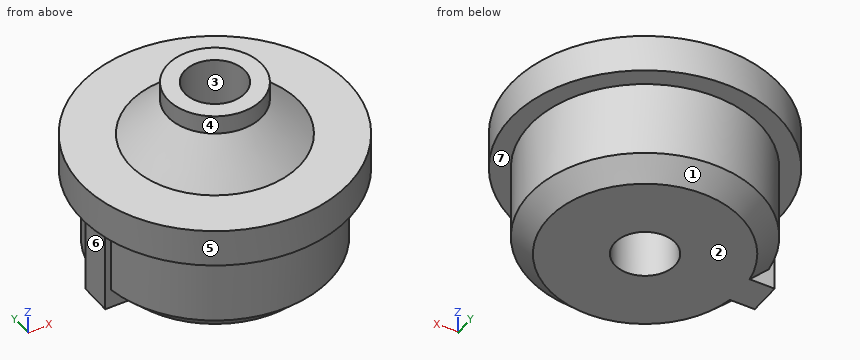
```python
from build123d import *

# Parameters (mm, degrees)
EXTRUDE_1_DEPTH     = 5
SKETCH_2_R          = 7.1
EXTRUDE_2_DEPTH     = 2
SKETCH_3_R          = 2.5
EXTRUDE_3_DEPTH     = 7
CHAMFER_1_SIZE      = 2
SKETCH_4_R          = 1.6
CUT_EXTRUDE_1_DEPTH = 30
CHAMFER_2_SIZE      = 1
MOVE_FACE_1_BY      = 4


with BuildPart() as part:
    # ｽｹｯﾁ1 → ﾎﾞｽ - 押し出し1 (new body)
    with BuildSketch(Plane.XY):
        with BuildLine():
            Line((-6.35, -0.875), (-6.036917674, -0.875))
            ThreePointArc((-6.036917674, -0.875), (6.1, 0), (-6.036917674, 0.875))
            Line((-6.036917674, 0.875), (-6.35, 0.875))
            Line((-6.35, 0.875), (-6.35, -0.875))
        make_face()
    extrude(amount=-EXTRUDE_1_DEPTH)

    # ｽｹｯﾁ2 → ﾎﾞｽ - 押し出し2 (add)
    with BuildSketch(Plane.XY):
        Circle(SKETCH_2_R)
    extrude(amount=EXTRUDE_2_DEPTH)

    # ｽｹｯﾁ3 → ﾎﾞｽ - 押し出し3 (add)
    with BuildSketch(Plane.XY.offset(2)):
        Circle(SKETCH_3_R)
    extrude(amount=EXTRUDE_3_DEPTH)

    # 面取り1
    chamfer_1_edges = [part.edges().sort_by_distance(p)[0] for p in [
        (-2.5, 0, 2),
    ]]
    chamfer(chamfer_1_edges, length=CHAMFER_1_SIZE)

    # ｽｹｯﾁ4 → ｶｯﾄ - 押し出し1 (cut)
    with BuildSketch(Plane.XY.offset(9)):
        Circle(SKETCH_4_R)
    extrude(amount=-CUT_EXTRUDE_1_DEPTH, mode=Mode.SUBTRACT)

    # 面取り2
    chamfer_2_edges = [part.edges().sort_by_distance(p)[0] for p in [
        (6.1, 0, -5),
    ]]
    chamfer(chamfer_2_edges, length=CHAMFER_2_SIZE)

    # Move Face 1: a face moved inward by 4.0
    extrude(part.faces().sort_by_distance((0, -2, 9))[0], amount=MOVE_FACE_1_BY, dir=(0, 0, -1), mode=Mode.SUBTRACT)


solid = part.part
```
Check sheet for the modelled part. Datum: model origin and axes. Units: mm. Face numbers are marked on the shaded views. A direction names the side the tool comes from. Give positions to 0.01 mm unless a question says otherwise; leave off trailing zeros. Order: outer loops, then holes, each group sorted by start corner. A loop starts at its lowest first (then second) coordinate and runs counter-clockwise, first axis right, second up. Notation, with made-up numbers: (53.25, -37) -> (60.25, -37) arc R28 ccw to (60.25, -6) -> close; hole circle Ø5 at (15, 46.25). An arc over 180 degrees is marked (long way). Return JSON: item names as keys, results as strings.
1. Cross-section at C-C, the plane z = 3.5. Record the cut outline in (x, y).
From the geometry:
{"outline": "circle Ø6 at (0, 0); hole circle Ø3.2 at (0, 0)"}
2. Material ranges on probe 1 along Y at (x, z) = (0, -2.75); probe 2 along Y at (x, z) = (-5.75, -4.5) (3 decimals); probe 3 along Z at (x, y) = (-0.5, -5), recorded low to high. Write a range as [from, to].
From the geometry:
{"probe 1": "[-6.1, -1.6], [1.6, 6.1]", "probe 2": "[-0.875, 0.875]", "probe 3": "[-5, 2]"}
3. Cross-section at A-A, the plane y = 0. Record the cut outline in (x, z), plus the area to 4 significant figures.
From the geometry:
{"outline": "(-7.1, 0) -> (-6.35, 0) -> (-6.35, -5) -> (-1.6, -5) -> (-1.6, 5) -> (-2.5, 5) -> (-2.5, 4) -> (-4.5, 2) -> (-7.1, 2) -> close; (1.6, -5) -> (5.1, -5) -> (6.1, -4) -> (6.1, 0) -> (7.1, 0) -> (7.1, 2) -> (4.5, 2) -> (2.5, 4) -> (2.5, 5) -> (1.6, 5) -> close", "area": "77.15 mm^2"}
4. Cross-section at B-B, the plane x = 0. Record the cut outline in (y, z), plus the area to 3 significant figures.
From the geometry:
{"outline": "(-7.1, 0) -> (-6.1, 0) -> (-6.1, -4) -> (-5.1, -5) -> (-1.6, -5) -> (-1.6, 5) -> (-2.5, 5) -> (-2.5, 4) -> (-4.5, 2) -> (-7.1, 2) -> close; (1.6, -5) -> (5.1, -5) -> (6.1, -4) -> (6.1, 0) -> (7.1, 0) -> (7.1, 2) -> (4.5, 2) -> (2.5, 4) -> (2.5, 5) -> (1.6, 5) -> close", "area": "75.4 mm^2"}
5. Set-up check for the marked faces 4, 5, 6 and 7: record each of +Z, -Z, +X, -X, +Y, -Y from which the full face is reachable in a straight line by a thin tool's end or side.
From the geometry:
{"face 4": "+Z", "face 5": "+Z, -Z", "face 6": "-Z, -X, +Y, -Y", "face 7": "-Z"}
6. Go/stop test with flat-tipped pins: P1, Ø1.5, axis at x = -3.5, z = -2, coming from the +Y side; P2, Ø0.7, axis at x = -5.5, z = -3.5, coming from the +Y side; P3, Ø1, axis at x = -0.5, z = -4, coming from the -Y side. Record where each tip stops, or that it passes through.
From the geometry:
{"P1": "y = 5.44", "P2": "y = 3.27", "P3": "y = -6.1"}
7. Mould release check, pull along Y, two halves, no side actions. Record for the marked faces 1, 2 and 3: +Y half, -Y half, draft (parallel to the pull), parting line (faces both ways), or undercut.
From the geometry:
{"face 1": "parting line", "face 2": "draft", "face 3": "undercut"}
8. Cross-section at D-D, the plane z = 1.75. Record the cut outline in (x, y), plus the area to 3 significant figures.
From the geometry:
{"outline": "circle Ø14.2 at (0, 0); hole circle Ø3.2 at (0, 0)", "area": "150 mm^2"}
